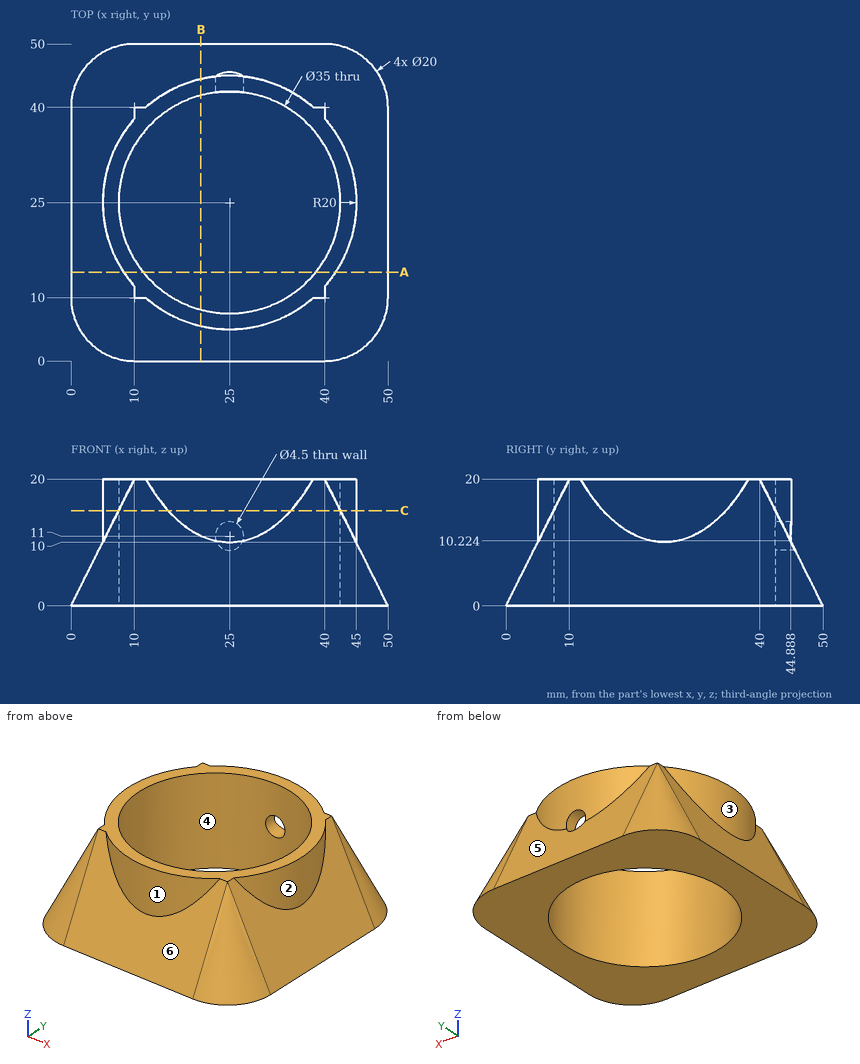
Check sheet for the drawn part. Datum: minimum x, y, z corner. Units: mm. A direction names the side the tool comes from. Give positions to 0.01 mm unless a question says otherwise; leave off trailing zeros. Write each loop counter-clockwise with the first axis right and the second up, starting at its lowest first coordinate (ties: lowest second). Pieces come first, ordered by that corner, then holes. Notation, with made-up numbers: M 48,-32 L 74,-32 A27 ccw 74,-13 Z; hole C 72.25,14.5 d11. An arc over 180 degrees is marked long. Write item = value, one per line.
(1) Material ranges on line 1 (Z direction, x = 25, y = 44); line 2 (Y direction, x = 24.5, z = 13.5); line 3 (Y direction, x = 20.5, z = 2.75) (1 decimal), recorded low to high.
Found:
line_1 = 0 to 8.75, 13.25 to 20
line_2 = 5.01 to 7.51, 42.49 to 44.99
line_3 = 1.4 to 8.1, 41.9 to 48.6
(2) Access from +Z, -Z, +X, -X, +Y, -Y to the whole of each face (thin tool, end or side, straight path). Record for the marked faces 1, 2 and 3.
Found:
face_1 = +Z, -Y
face_2 = +Z, +X
face_3 = +Z, -X
(3) Go/stop test with flat-tipped pins: pin 1 Ø2 at (x, z) = (26, 5.5) entering from +Y; pin 2 Ø3 at (y, z) = (28, 8) entering from -X; pin 3 Ø5 at (y, z) = (20, 17.5) entering from -X; pin 4 Ø21 at (x, y) = (25, 25) entering from -Z. Record where each tip stops, or that it passes through.
Found:
pin_1 = 47.75
pin_2 = 3.25
pin_3 = 5.16
pin_4 = through
(4) Sectioned sample at C-C (z = 15). Record the cut outline in (x, y).
Found:
outline = M 7.5,10 A2.5 ccw 10,7.5 L 15.32,7.5 A20 ccw 34.68,7.5 L 40,7.5 A2.5 ccw 42.5,10 L 42.5,15.32 A20 ccw 42.5,34.68 L 42.5,40 A2.5 ccw 40,42.5 L 34.68,42.5 A20 ccw 15.32,42.5 L 10,42.5 A2.5 ccw 7.5,40 L 7.5,34.68 A20 ccw 7.5,15.32 Z; hole C 25,25 d35
(5) Draft check along Y on the marked faces 4, 5 and 6. Enter one of: released by +Y, released by -Y, zero draft, split by the parting line, or undercut.
Found:
face_4 = undercut
face_5 = released by +Y
face_6 = released by -Y
(6) Sectioned sample at A-A (y = 14). Record the cut outline in (x, z).
Found:
outline = M 0,0 L 11.39,0 L 11.39,20 L 8.3,20 L 8.3,16.59 Z; M 38.61,0 L 50,0 L 41.7,16.59 L 41.7,20 L 38.61,20 Z
(7) Sectioned sample at B-B (x = 20.5). Record the cut outline in (y, z) (1 decimal).
Found:
outline = M 0,0 L 8.1,0 L 8.1,20 L 5.5,20 L 5.5,11 Z; M 41.9,0 L 50,0 L 44.5,11 L 44.5,20 L 41.9,20 Z
